```python
from build123d import *

# Parameters (mm, degrees)
F1_DEPTH = 42
F3_DEPTH = 16.5


with BuildPart() as f1:
    # F0 (on Front) → F1 (new body)
    with BuildSketch(Plane.XZ):
        with BuildLine():
            Line((0, 22), (0, 13.536567))
            Line((0, 13.536567), (0, 0))
            ThreePointArc((0, 0), (-6, -6), (-12, 0))
            Line((-12, 0), (-12, 3.663141))
            ThreePointArc((-12, 3.663141), (-13.5, 5.163141), (-15, 3.663141))
            Line((-15, 3.663141), (-15, 0))
            ThreePointArc((-15, 0), (-13.649713, -4.741507), (-10.004025, -8.060259))
            Line((-10.004025, -8.060259), (-8.524168, -8.638783))
            ThreePointArc((-8.524168, -8.638783), (-0.601737, -7.201302), (3, 0))
            Line((3, 0), (3, 22))
            ThreePointArc((3, 22), (5.843606, 23.509868), (7.25, 20.613689))
            Line((7.25, 20.613689), (7.25, 16.640851))
            ThreePointArc((7.25, 16.640851), (8.233139, 25.554439), (0, 22))
        make_face()
        with BuildLine():
            Line((-8.524168, -8.638783), (-10.004025, -8.060259))
            ThreePointArc((-10.004025, -8.060259), (-9.276889, -8.382243), (-8.524168, -8.638783))
        make_face()
    extrude(amount=F1_DEPTH)

    # F2 (on face) → F3 (cut, symmetric)
    with BuildSketch(Plane(origin=(0, 0, 0), x_dir=(0, -1, 0), z_dir=(-1, 0, 0))):
        Polygon((7.5, 9), (7.5, -16.111853), (34.5, -18.625535), (34.5, 9), align=None)
    extrude(amount=F3_DEPTH, both=True, mode=Mode.SUBTRACT)


solid = f1.part
```
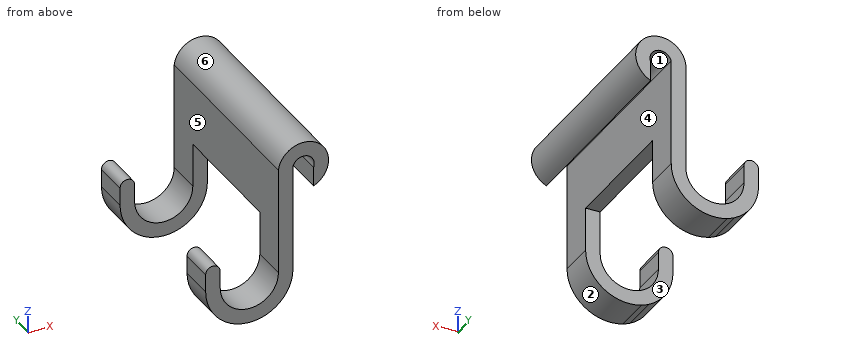
Read the model definition and answer for the solid it produces. Units are mm, in the model's axes. Face numbers are marked on the shaded views. A direction names the side the tool comes from. Round coordinates to 2 decimals unless told otherwise and drop trailing zeros. Write each loop counter-clockwise with the first axis right and the second up, starting at its lowest first coordinate (ties: lowest second). Pieces come first, ordered by that corner, then holes. Notation, with made-up numbers: (40, -1) -> (88, -1) arc R34 cw to (88, 35) -> close; hole circle Ø2 at (37.25, 10.5). An arc over 180 degrees is marked (long way). Answer in a Markdown table with one row per item. Add a question column.
1) Find section C-C, the plane z = 18. Determine the outline of the cut face in (x, y), and give its area (3 significant figures).
2) Find section B-B, the plane y = -36.5. Determine the outline of the cut face in (x, z), and give its area (3 significant figures).
3) Which of the six approach directions +Z, -Z, +X, -X, +Y, -Y give full straight-line access (tool end or side, diameter ignored) to the marked faces 4, 5 and 6?
4) Find section D-D, the plane x = 5.15. Determine the outline of the cut face in (y, z), and give its area (3 significant figures).
5) Consider line 1 (Y direction, x = -11.75, z = -2); line 2 (X direction, y = -13.5, z = 14); line 3 (X direction, y = -11, z = 17). Determine where each line is inside the solid, lowest interval first.
6) Determine the mould class of the marked faces 1, 2 and 3 for opening direction X: pulls with the +X half, pulls with the -X half, needs draft (parallel to the pull), parting line crosses it, or undercut.
7) Find section A-A, the plane x = -3.5. Determine the outline of the cut face in (y, z).
8) Given P1, Ø10, axis at y = -26, z = 9, coming from the +X side; P2, Ø11, axis at y = -21.5, z = 13.5, coming from the -X side; P3, Ø2.5, axis at x = 1.5, y = -23, coming from the -Z side; P4, Ø5, axis at x = -4.5, y = -14.5, coming from the -Z side, each flat-ended and moving along its own axis, determine where each tip first touches the part or whether it passes through.
Findings below:
| question | item | result |
|---|---|---|
| 1 | outline | (0, -42) -> (3, -42) -> (3, 0) -> (0, 0) -> close; (7.25, -42) -> (9.08, -42) -> (9.08, 0) -> (7.25, 0) -> close |
| 1 | area | 203 mm² |
| 2 | outline | (-15, 0) arc R9 ccw to (-10, -8.06) arc R9 ccw to (-8.52, -8.64) arc R9 ccw to (3, 0) -> (3, 22) arc R2.24 cw (long way) to (7.25, 20.61) -> (7.25, 16.64) arc R5.19 ccw (long way) to (0, 22) -> (0, 0) arc R6 cw to (-12, 0) -> (-12, 3.66) arc R1.5 ccw to (-15, 3.66) -> close |
| 2 | area | 194 mm² |
| 3 | face 4 | -Z, +Y, -Y |
| 3 | face 5 | +Z, +Y, -Y |
| 3 | face 6 | +Y, -Y |
| 4 | outline | (-42, 23.62) -> (0, 23.62) -> (0, 26.57) -> (-42, 26.57) -> close |
| 4 | area | 124 mm² |
| 5 | line 1 | -42 to -34.5, -7.5 to 0 |
| 5 | line 2 | 0 to 3 |
| 5 | line 3 | 0 to 3, 7.25 to 7.92 |
| 6 | face 1 | undercut |
| 6 | face 2 | parting line crosses it |
| 6 | face 3 | needs draft |
| 7 | outline | (-42, -8.65) -> (-34.5, -8.65) -> (-34.5, -5.45) -> (-42, -5.45) -> close; (-7.5, -8.65) -> (0, -8.65) -> (0, -5.45) -> (-7.5, -5.45) -> close |
| 8 | P1 | x = 3 |
| 8 | P2 | x = 0 |
| 8 | P3 | z = 9 |
| 8 | P4 | through |
